Design review of the part built by this model. Coordinates are the model's own, in mm. Round coordinates to 2 decimals unless told otherwise and drop trailing zeros. Order: outer loops, then holes, each group sorted by start corner. A loop starts at its lowest first (then second) coordinate and runs counter-clockwise, first axis right, second up. Notation, with made-up numbers: M -2.5,-34 L 21.5,-34 A8 ccw 21.5,-28 Z; hole C -21,56.5 d6. An arc over 180 degrees is marked long. Use a Markdown table: item, result. Add a question column.
(1) Take a section at C-C (y = -71.5). Write out the cut boundary in (x, z), then the cut area to 3 significant figures.
(2) Take a section at A-A (z = 7). Write out the cut boundary in (x, y).
(3) For pin 1 (10 mm diameter, centred on x = -46.5, z = 9, fed in from -Y); pin 2 (1 mm diameter, centred on y = 75, z = 17, fed in from +X); pin 3 (1 mm diameter, centred on x = -33, z = 8.5, fed in from -Y), all flat-tipped, find the tip position at first contact; note any pin that passes through.
(4) Take a section at B-B (x = 54). Write out the cut boundary in (y, z), then the cut area to 3 significant figures.
(5) To check wall thickness, follow probe 1 along Y at (x, z) = (-47, 12.75); probe 2 along Y at (x, z) = (30, 4); probe 3 along X at (y, z) = (-67, 6.5). State the ranges of each line that lie inside material, in increasing order. Write a range as from..to.
```python
from build123d import *

# Parameters (mm, degrees)
F0_W     = 57.912
F0_H     = 32.6462263381
F0_W_2   = 36.5589186821
F0_H_2   = 131.572
F1_DEPTH = 19.05


with BuildPart() as f1:
    # F0 (on Top) → F1 (new body)
    with BuildSketch(Plane.XY):
        with Locations((0, 82.109113169)):
            Rectangle(F0_W, F0_H)
        with Locations((-47.2354593411, 0)):
            Rectangle(F0_W_2, F0_H_2)
        Polygon((-28.956, 65.786), (-28.956, 98.4322263381), (-65.5149186821, 65.786), align=None)
        Rectangle(F0_W, F0_H_2)
        with Locations((47.2354593411, 0)):
            Rectangle(F0_W_2, F0_H_2)
        Polygon((65.5149186821, 65.786), (28.956, 98.4322263381), (28.956, 65.786), align=None)
        Polygon((65.5149186821, -65.786), (28.956, -65.786), (28.956, -98.4322263381), align=None)
        with Locations((0, -82.109113169)):
            Rectangle(F0_W, F0_H)
        Polygon((-28.956, -98.4322263381), (-28.956, -65.786), (-65.5149186821, -65.786), align=None)
    extrude(amount=F1_DEPTH)


solid = f1.part
```
Verdict:
| question | item | result |
|---|---|---|
| 1 | outline | M -59.12,0 L 59.12,0 L 59.12,19.05 L -59.12,19.05 Z |
| 1 | area | 2,250 mm^2 |
| 2 | outline | M -65.51,-65.79 L -28.96,-98.43 L 28.96,-98.43 L 65.51,-65.79 L 65.51,65.79 L 28.96,98.43 L -28.96,98.43 L -65.51,65.79 Z |
| 3 | pin 1 | stops at y = -87.23 |
| 3 | pin 2 | stops at x = 55.76 |
| 3 | pin 3 | stops at y = -95.27 |
| 4 | outline | M -76.07,0 L 76.07,0 L 76.07,19.05 L -76.07,19.05 Z |
| 4 | area | 2,900 mm^2 |
| 5 | probe 1 | y = -82.32..82.32 |
| 5 | probe 2 | y = -97.5..97.5 |
| 5 | probe 3 | x = -64.16..64.16 |
